Check sheet for the modelled part. Datum: model origin and axes. Units: mm. Face numbers are marked on the shaded views. Round coordinates to 2 decimals unless told otherwise and drop trailing zeros. Write each loop counter-clockwise with the first axis right and the second up, starting at its lowest first coordinate (ties: lowest second). Pieces come first, ordered by that corner, then holes.
Item 1: Material ranges on line 1 along Z through (x, y) = (2, 2); line 2 along Z through (x, y) = (1, 1.5); line 3 along X through (y, z) = (7.75, 3.5), recorded low to high.
Item 2: Section check D-D, the plane z = 31. Record the cut outline in (x, y).
Item 3: Release check for a two-part mould opening along Z. For the marked faces 1, 2 and 3 record: pulls with the +Z half, pulls with the -Z half, needs draft (parallel to the pull), parting line crosses it, or undercut.
Item 4: Section check B-B, the plane z = 6.5. Record the cut outline in (x, y).
Item 5: Section check A-A, the plane y = 4. Record the cut outline in (x, z), plus the area to 3 significant figures.
Item 6: Section check C-C, the plane x = 0.5. Record the cut outline in (y, z), plus the area to 3 significant figures.
Item 7: Depth check by flat-ended pin: pin 1 (1 mm diameter, centred on x = 6, y = 1.5, fed in from +Z); pin 2 (1 mm diameter, centred on x = -5, y = 1.5, fed in from -Z); pin 3 (1 mm diameter, centred on x = 3.5, y = 5, fed in from -Z). Enter the tip coordinate at first touch or a pass-through.
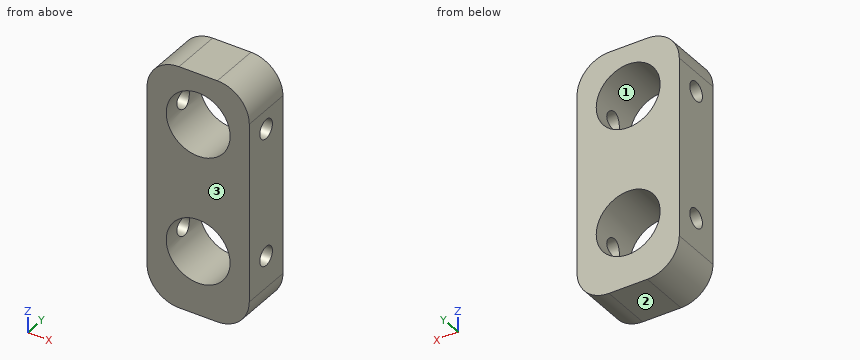
from build123d import *

# Parameters (mm, degrees)
SKETCH1_R           = 5
BOSS_EXTRUDE1_DEPTH = 8
SKETCH2_R           = 1.5
CUT_EXTRUDE1_DEPTH  = 17


with BuildPart() as part:
    # Sketch1 → Boss-Extrude1 (new body)
    with BuildSketch(Plane(origin=(0, 0, 0), x_dir=(1, 0, 0), z_dir=(0, 1, 0))):
        with BuildLine():
            Line((-2.673601855, -35.379310345), (3.326398145, -35.379310345))
            ThreePointArc((3.326398145, -35.379310345), (6.861932051, -33.914844251), (8.326398145, -30.379310345))
            Line((8.326398145, -30.379310345), (8.326398145, -2.379310345))
            ThreePointArc((8.326398145, -2.379310345), (6.861932051, 1.156223561), (3.326398145, 2.620689655))
            Line((3.326398145, 2.620689655), (-2.673601855, 2.620689655))
            ThreePointArc((-2.673601855, 2.620689655), (-6.20913576, 1.156223561), (-7.673601855, -2.379310345))
            Line((-7.673601855, -2.379310345), (-7.673601855, -30.379310345))
            ThreePointArc((-7.673601855, -30.379310345), (-6.20913576, -33.914844251), (-2.673601855, -35.379310345))
        make_face()
        with Locations((0.326398145, -27.379310345)):
            Circle(SKETCH1_R, mode=Mode.SUBTRACT)
        with Locations((0.326398145, -7.379310345)):
            Circle(SKETCH1_R, mode=Mode.SUBTRACT)
    extrude(amount=BOSS_EXTRUDE1_DEPTH)

    # Sketch2 → Cut-Extrude1 (cut, through all)
    with BuildSketch(Plane(origin=(8.326398145, 0, 0), x_dir=(0, 0, -1), z_dir=(1, 0, 0))):
        with Locations((-27.379310345, 4)):
            Circle(SKETCH2_R)
        with Locations((-7.379310345, 4)):
            Circle(SKETCH2_R)
    extrude(amount=-CUT_EXTRUDE1_DEPTH, mode=Mode.SUBTRACT)


solid = part.part
Values found:
1. line 1: z = -2.62 to 2.67, 12.09 to 22.67, 32.09 to 35.38
1. line 2: z = -2.62 to 2.42, 12.33 to 22.42, 32.33 to 35.38
1. line 3: x = -7.67 to -2.83, 3.48 to 8.33
2. outline: (-7.63, 0) - (-3.12, 0) - (-3.12, 8) - (-7.63, 8) - close; (3.77, 0) - (8.29, 0) - (8.29, 8) - (3.77, 8) - close
3. face 1: undercut
3. face 2: pulls with the -Z half
3. face 3: needs draft
4. outline: (-7.67, 0) - (-4.6, 0) - (-4.6, 2.78) - (-7.67, 2.78) - close; (-7.67, 5.22) - (-4.6, 5.22) - (-4.6, 8) - (-7.67, 8) - close; (5.25, 0) - (8.33, 0) - (8.33, 2.78) - (5.25, 2.78) - close; (5.25, 5.22) - (8.33, 5.22) - (8.33, 8) - (5.25, 8) - close
5. outline: (-7.67, 2.38) arc R5 ccw to (-2.67, -2.62) - (3.33, -2.62) arc R5 ccw to (8.33, 2.38) - (8.33, 5.88) - (5.1, 5.88) arc R5 cw to (-4.44, 5.88) - (-7.67, 5.88) - close; (-7.67, 8.88) - (-4.44, 8.88) arc R5 cw to (5.1, 8.88) - (8.33, 8.88) - (8.33, 25.88) - (5.1, 25.88) arc R5 cw to (-4.44, 25.88) - (-7.67, 25.88) - close; (-7.67, 28.88) - (-4.44, 28.88) arc R5 cw to (5.1, 28.88) - (8.33, 28.88) - (8.33, 30.38) arc R5 ccw to (3.33, 35.38) - (-2.67, 35.38) arc R5 ccw to (-7.67, 30.38) - close
5. area: 393 mm2
6. outline: (0, -2.62) - (8, -2.62) - (8, 2.38) - (0, 2.38) - close; (0, 12.38) - (8, 12.38) - (8, 22.38) - (0, 22.38) - close; (0, 32.38) - (8, 32.38) - (8, 35.38) - (0, 35.38) - close
6. area: 144 mm2
7. pin 1: stops at z = 34.88
7. pin 2: stops at z = -2.28
7. pin 3: stops at z = -2.62
